Verification items for the finished model (mm, model axes). Face numbers are marked on the shaded views. A direction names the side the tool comes from. Round coordinates to 2 decimals unless told otherwise and drop trailing zeros. Write each loop counter-clockwise with the first axis right and the second up, starting at its lowest first coordinate (ties: lowest second). Pieces come first, ordered by that corner, then holes. Notation, with made-up numbers: M 18.5,60 L 63.5,60 A22 cw 63.5,98 Z; hole C -7,74.25 d11. An arc over 180 degrees is marked long. One line per item, written item: value. Start each with the question number.
Item 1: Section check D-D, the plane y = 9. State how many separate pieces and enclosed holes the cut face has, then the cut area to 3 significant figures.
Item 2: Gauge pin test, flat ends, axial feed: pin 1 (6.5 mm diameter, centred on y = 10, z = 30.2, fed in from -X); pin 2 (8 mm diameter, centred on x = 10.5, y = 4, fed in from +Z). Record the tip position at first contact, or that the pin passes through.
Item 3: Draft check along Y on the marked faces 1, 2 and 3. Enter one of: +Y half, -Y half, draft (parallel to the pull), parting line (faces both ways), or undercut.
Item 4: Section check C-C, the plane y = 14.5. Record the cut outline in (x, z).
Item 5: Section check B-B, the plane x = 13. Record the cut outline in (y, z), then the cut area to 3 significant figures.
Item 6: Thickness scan on probe 1 along Y at (x, z) = (18, -1); probe 2 along Y at (x, z) = (20, -1); probe 3 along X at (y, z) = (3.75, 12). Record the ranges inside material, lowest first. Write a range as from..to.
Item 7: Tool access check on the marked faces 4 and 5. Record the directions out of +Z, -Z, +X, -X, +Y, -Y that give a thin tool (end or side, any length) a straight path to the whole face; none if there is none.
Item 8: Section check A-A, the plane x = 18. Record the cut outline in (y, z), then the cut area to 3 significant figures.
from build123d import *

# Parameters (mm, degrees)
ESQUISSE1_W             = 3
ESQUISSE1_H             = 20
BOSS_EXTRU_1_DEPTH      = 41.27
ESQUISSE1_3_W           = 36
ESQUISSE1_3_H           = 20
BOSS_EXTRU_2_DEPTH      = 3
ESQUISSE3_R             = 1.5
ESQUISSE3_R_2           = 2.5
ENL_V_MAT_EXTRU_2_DEPTH = 85
CONG_2_R                = 2
CONG_3_R                = 10
ESQUISSE7_R             = 1.5
ESQUISSE7_R_2           = 2.5
ENL_V_MAT_EXTRU_3_DEPTH = 10


with BuildPart() as part:
    # Esquisse1 → Boss.-Extru.1 (new body)
    with BuildSketch(Plane.XY):
        with Locations((34.5, 10)):
            Rectangle(ESQUISSE1_W, ESQUISSE1_H)
    extrude(amount=BOSS_EXTRU_1_DEPTH)

    # Esquisse1<3> → Boss.-Extru.2 (add)
    with BuildSketch(Plane.XY):
        with Locations((18, 10)):
            Rectangle(ESQUISSE1_3_W, ESQUISSE1_3_H)
    extrude(amount=-BOSS_EXTRU_2_DEPTH)

    # Esquisse3 → Enlèv. mat.-Extru.2 (cut)
    with BuildSketch(Plane(origin=(36, 0, 0), x_dir=(0, 0, -1), z_dir=(1, 0, 0))):
        with Locations((-30.197874881, 15)):
            Circle(ESQUISSE3_R)
        with Locations((-30.197874881, 5)):
            Circle(ESQUISSE3_R)
        with Locations((-35.197874881, 10)):
            Circle(ESQUISSE3_R)
        with Locations((-25.197874881, 10)):
            Circle(ESQUISSE3_R)
        with Locations((-30.197874881, 10)):
            Circle(ESQUISSE3_R_2)
    extrude(amount=-ENL_V_MAT_EXTRU_2_DEPTH, mode=Mode.SUBTRACT)

    # Congé2
    cong_2_edges = [part.edges().sort_by_distance(p)[0] for p in [
        (33, 10, 0),
    ]]
    fillet(cong_2_edges, radius=CONG_2_R)

    # Congé3
    cong_3_edges = [part.edges().sort_by_distance(p)[0] for p in [
        (0, 20, -1.5),
        (0, 0, -1.5),
        (34.5, 20, 41.27),
        (34.5, 0, 41.27),
    ]]
    fillet(cong_3_edges, radius=CONG_3_R - 0.0001)  # a hair under: the kernel refuses the full size

    # Esquisse7 → Enlèv. mat.-Extru.3 (cut)
    with BuildSketch(Plane(origin=(0, 0, -3), x_dir=(-1, 0, 0), z_dir=(0, 0, -1))):
        with Locations((-23, 10)):
            Circle(ESQUISSE7_R)
        with Locations((-18, 15)):
            Circle(ESQUISSE7_R)
        with Locations((-13, 10)):
            Circle(ESQUISSE7_R)
        with Locations((-18, 5)):
            Circle(ESQUISSE7_R)
        with Locations((-18, 10)):
            Circle(ESQUISSE7_R_2)
    extrude(amount=-ENL_V_MAT_EXTRU_3_DEPTH, mode=Mode.SUBTRACT)


solid = part.part
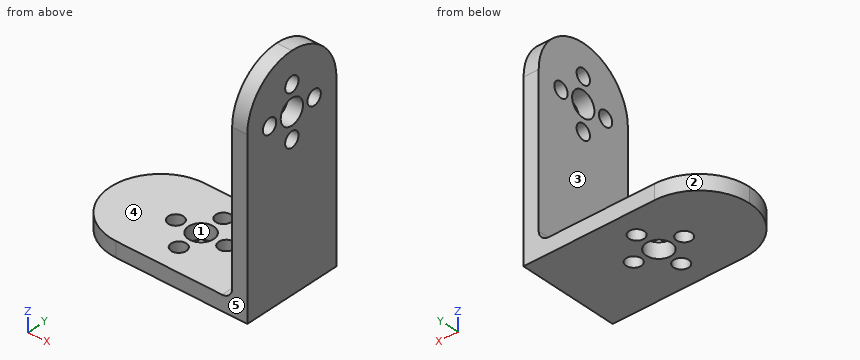
Response values:
1. separate pieces: 7
1. enclosed holes: 0
1. area: 178 mm2
2. pin 1: stops at x = 33
2. pin 2: stops at z = 0
3. face 1: undercut
3. face 2: +Y half
3. face 3: draft
4. outline: M 1.07,-3 L 16.59,-3 L 16.59,0 L 1.07,0 Z; M 19.41,-3 L 36,-3 L 36,28.78 L 33,28.78 L 33,2 A2 cw 31,0 L 19.41,0 Z; M 33,31.61 L 36,31.61 L 36,40.2 L 33,40.2 Z
5. outline: M 0,-3 L 8.5,-3 L 8.5,0 L 0,0 Z; M 11.5,-3 L 20,-3 L 20,0 L 11.5,0 Z
5. area: 51.0 mm2
6. probe 1: y = 0..3.5, 6.5..7.5, 12.5..13.5, 16.5..20
6. probe 2: y = 0..8.5, 11.5..20
6. probe 3: x = 33..36
7. face 4: +Z, -X, +Y, -Y
7. face 5: +Z, -Z, +X, -X, -Y
8. outline: M 0,-3 L 3.5,-3 L 3.5,0 L 0,0 Z; M 6.5,-3 L 7.5,-3 L 7.5,0 L 6.5,0 Z; M 12.5,-3 L 13.5,-3 L 13.5,0 L 12.5,0 Z; M 16.5,-3 L 20,-3 L 20,0 L 16.5,0 Z
8. area: 27.0 mm2
